Can you work these out from the model? Positions are in its coordinate system, mm. Face numbers are marked on the shaded views. A direction names the side the tool comes from. Round coordinates to 2 decimals unless told otherwise and drop trailing zeros. Order: outer loops, then holes, each group sorted by start corner. A loop starts at its lowest first (then second) coordinate and runs counter-clockwise, first axis right, second up. Notation, with made-up numbers: (19.5, 85) -> (59.5, 85) arc R8 cw to (59.5, 89) -> close; hole circle Ø7 at (33, -39.75). An arc over 180 degrees is marked (long way). Use a Markdown table: item, result. Add a question column.
Q1. I'm going to push flat-ended pins straight in: pin 1 Ø4.5 at (y, z) = (-3, 1.5) entering from -X; pin 2 Ø10 at (x, y) = (-15.35, 0) entering from +Z; pin 3 Ø4 at (y, z) = (8.5, 5.5) entering from +X. Where does each tip first touch, or does it pass through?
Q2. I need wall thicknesses on line 1 along Y through (x, z) = (0, 2.75); line 2 along Z through (x, y) = (22.5, -7); line 3 along Y through (x, z) = (-10, 10.25). Which ranges of each line are inside material? Lowest first, please. Write a range as [from, to].
Q3. We'd pull the mould along Y, two halves only. Please class the marked faces 6, 7 and 8: +Y half, -Y half, draft (parallel to the pull), parting line (faces both ways), or undercut.
Q4. If we section it at B-B on x = 13.5: List the corners of the cut face in (y, z) for me, plus the area to 3 significant figures.
Q5. If we section it at C-C on y = -16.5: List the corners of the cut face in (x, z) for me.
Q6. For the marked faces 1, 2, 3, 4 and 5, which set-ups out of +Z, -Z, +X, -X, +Y, -Y let a thin tool reach every point of the face, with its end or its side?
Q7. If we section it at D-D on z = 5: List the corners of the cut face in (x, y) for me.
Q8. If we section it at A-A on x = 0: List the corners of the cut face in (y, z) for me.
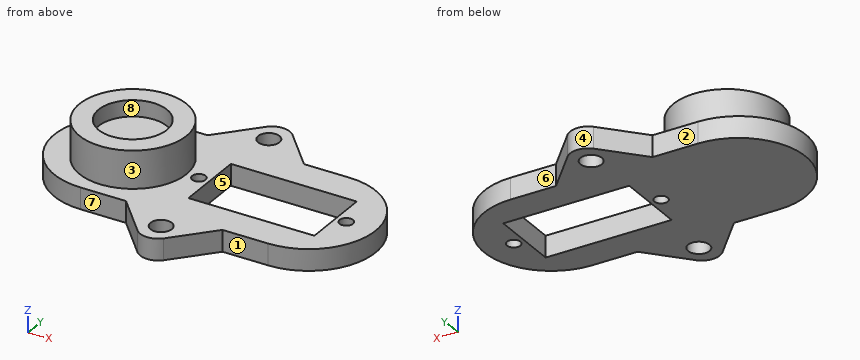
```python
from build123d import *

# Parameters (mm, degrees)
SKETCH1_R           = 2
SKETCH1_R_2         = 1.25
SKETCH1_W           = 23.5
SKETCH1_H           = 13
BOSS_EXTRUDE1_DEPTH = 4
SKETCH3_R           = 10
BOSS_EXTRUDE2_DEPTH = 7
SKETCH4_R           = 6.377506195
CUT_EXTRUDE1_DEPTH  = 3


with BuildPart() as part:
    # Sketch1 → Boss-Extrude1 (new body)
    with BuildSketch(Plane.XY):
        with BuildLine():
            Line((-9, 12.5), (-2.401010284, 19.772380391))
            ThreePointArc((-2.401010284, 19.772380391), (0, 20.766911414), (2.401010284, 19.772380391))
            Line((2.401010284, 19.772380391), (9, 12.5))
            Line((9, 12.5), (17.5, 12.5))
            ThreePointArc((17.5, 12.5), (30, 0), (17.5, -12.5))
            Line((17.5, -12.5), (9, -12.5))
            Line((9, -12.5), (2.401010284, -19.772380391))
            ThreePointArc((2.401010284, -19.772380391), (0, -20.766911414), (-2.401010284, -19.772380391))
            Line((-2.401010284, -19.772380391), (-9, -12.5))
            Line((-9, -12.5), (-17.5, -12.5))
            ThreePointArc((-17.5, -12.5), (-30, 0), (-17.5, 12.5))
            Line((-17.5, 12.5), (-9, 12.5))
        make_face()
        with Locations((0, 16.5)):
            Circle(SKETCH1_R, mode=Mode.SUBTRACT)
        with Locations((0, -16.5)):
            Circle(SKETCH1_R, mode=Mode.SUBTRACT)
        with Locations((-3, 0)):
            Circle(SKETCH1_R_2, mode=Mode.SUBTRACT)
        with Locations((24.5, 0)):
            Circle(SKETCH1_R_2, mode=Mode.SUBTRACT)
        with Locations((10.75, 0)):
            Rectangle(SKETCH1_W, SKETCH1_H, mode=Mode.SUBTRACT)
    extrude(amount=BOSS_EXTRUDE1_DEPTH)

    # Sketch3 → Boss-Extrude2 (add)
    with BuildSketch(Plane.XY.offset(4)):
        with Locations((-15.3, 0)):
            Circle(SKETCH3_R)
    extrude(amount=BOSS_EXTRUDE2_DEPTH)

    # Sketch4 → Cut-Extrude1 (cut)
    with BuildSketch(Plane.XY.offset(11)):
        with Locations((-15.35, 0)):
            Circle(SKETCH4_R)
    extrude(amount=-CUT_EXTRUDE1_DEPTH, mode=Mode.SUBTRACT)


solid = part.part
```
Answer below:
| question | item | result |
|---|---|---|
| 1 | pin 1 | x = -29.98 |
| 1 | pin 2 | z = 8 |
| 1 | pin 3 | x = 27.73 |
| 2 | line 1 | [-20.77, -18.5], [-14.5, -6.5], [6.5, 14.5], [18.5, 20.77] |
| 2 | line 2 | [0, 4] |
| 2 | line 3 | [-8.48, -3.47], [3.47, 8.48] |
| 3 | face 6 | +Y half |
| 3 | face 7 | -Y half |
| 3 | face 8 | undercut |
| 4 | outline | (-12.5, 0) -> (-6.5, 0) -> (-6.5, 4) -> (-12.5, 4) -> close; (6.5, 0) -> (12.5, 0) -> (12.5, 4) -> (6.5, 4) -> close |
| 4 | area | 48.0 mm² |
| 5 | outline | (-5.37, 0) -> (-2, 0) -> (-2, 4) -> (-5.37, 4) -> close; (2, 0) -> (5.37, 0) -> (5.37, 4) -> (2, 4) -> close |
| 6 | face 1 | +Z, -Z, +X, -Y |
| 6 | face 2 | +Z, -Z, -X, +Y |
| 6 | face 3 | +Z |
| 6 | face 4 | +Z, -Z, +Y |
| 6 | face 5 | +Z, -Z |
| 7 | outline | circle Ø20 at (-15.3, 0) |
| 8 | outline | (-20.77, 0) -> (-18.5, 0) -> (-18.5, 4) -> (-20.77, 4) -> close; (-14.5, 0) -> (-6.5, 0) -> (-6.5, 4) -> (-14.5, 4) -> close; (6.5, 0) -> (14.5, 0) -> (14.5, 4) -> (6.5, 4) -> close; (18.5, 0) -> (20.77, 0) -> (20.77, 4) -> (18.5, 4) -> close |
